Solid Edge part; units mm, degrees
sketch "Sketch1" plane through (0, 0, 0) normal (0, 0, 1) x (1, 0, 0)
  line L0 (0, 32.5) -> (0, 6.5)
  line L1 (13, 6.5) -> (13, 32.5)
  arc A0 (13, 6.5) -> (0, 6.5) centre (6.5, 6.5) cw
  arc A1 (0, 32.5) -> (13, 32.5) centre (6.5, 32.5) cw
extrude "Protrusion1" add sketch "Sketch1" along normal blind 6.5
sketch "Sketch2" plane through (6.5, 0, 0) normal (1, 0, 0) x (0, 1, 0)
  line L0 (3.5, 5.5) -> (3.5, 6.5)
  line L1 (3.5, 6.5) -> (6.5, 6.5)
  line L2 (6.5, 1) -> (6.5, 6.5)
  line L3 (3.5, 1) -> (6.5, 1)
  line L4 (3.5, 1) -> (2.6811, 3.25)
  line L5 (3.5, 5.5) -> (2.6811, 3.25)
revolve "RevolvedCutout1" cut sketch "Sketch2" angle 360 about axis through (6.5, 6.5, 1) along (0, 0, 1)
chamfer "Chaflán_38" distance 0.75 angle 45 1 edges at (6.5, 3.5, 6.5)
pattern_linear "Pattern1" count 3 spacing 13 along (0, 1, 0) of "RevolvedCutout1", "Chaflán_38"
chamfer "Chaflán_39" distance 1.5 angle 45 8 edges at (13, 19.5, 6.5) (6.5, 0, 6.5) (0, 19.5, 6.5) (6.5, 39, 6.5) (13, 19.5, 0) (6.5, 0, 0) (0, 19.5, 0) (6.5, 39, 0)
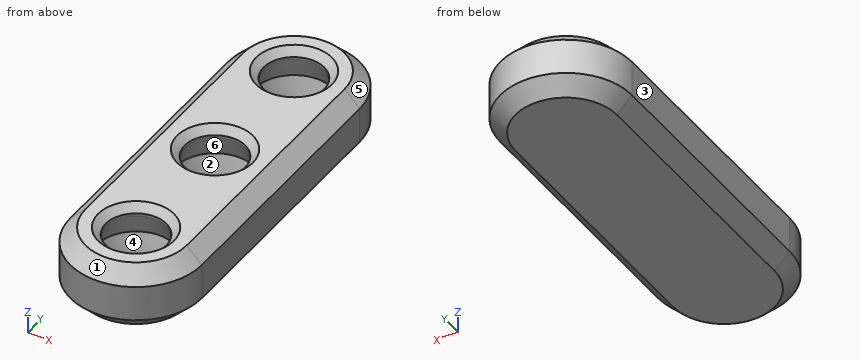
Can you work these out from the model? Positions are in its coordinate system, mm. Face numbers are marked on the shaded views. A direction names the side the tool comes from. Coordinates: 2 decimals unless noted, no trailing zeros. Write each loop counter-clockwise with the first axis right and the second up, starting at its lowest first coordinate (ties: lowest second). Pieces come first, ordered by that corner, then holes. Notation, with made-up numbers: M -29,-18 L 7,-18 A27 ccw 7,11 Z; hole C 55,69.25 d5. An arc over 180 degrees is marked long. Use one line per item in the form item = value.
Q1. I need wall thicknesses on line 1 along Y through (x, z) = (8.5, 4.5); line 2 along Y through (x, z) = (5.25, 6); line 3 along X through (y, z) = (32.5, 5.7). Which ranges of each line are inside material? Lowest first, please. Write a range as from..to.
Model answer:
line_1 = 0.32..3.8, 9.2..16.8, 22.2..29.8, 35.2..38.68
line_2 = 1.14..3.5, 9.5..16.5, 22.5..29.5, 35.5..37.86
line_3 = 0.7..3.5, 9.5..12.3
Q2. For P1, Ø3, axis at x = 5.5, y = 31, coming from the +Z side; P2, Ø3, axis at x = 4.5, z = 0.5, coming from the -Y side; P3, Ø1.8, axis at x = 6, y = 5, coming from the +Z side, each with a flat end and sliding along its axis, tell me the tip position at first contact or that it passes through.
Model answer:
P1 = 6.05
P2 = 0.06
P3 = 1
Q3. For the marked faces 5 and 6, which set-ups out of +Z, -Z, +X, -X, +Y, -Y let a thin tool reach every point of the face, with its end or its side?
Model answer:
face_5 = +Z, +Y
face_6 = none
Q4. If we section it at A-A (y = 19.5): Write out the boundary of the cut face in (x, z), then the cut area to 3 significant figures.
Model answer:
outline = M 0,1.5 L 1.5,0 L 11.5,0 L 13,1.5 L 13,5 L 11.5,6.5 L 10.25,6.5 L 9.5,5.75 L 9.5,5.5 L 10.32,3.25 L 9.5,1 L 3.5,1 L 2.68,3.25 L 3.5,5.5 L 3.5,5.75 L 2.75,6.5 L 1.5,6.5 L 0,5 Z
area = 42.8 mm^2
Q5. If we section it at B-B (z = 4.25): Write out the boundary of the cut face in (x, y).
Model answer:
outline = M 0,6.5 A6.5 ccw 13,6.5 L 13,32.5 A6.5 ccw 0,32.5 Z; hole C 6.5,6.5 d6.91; hole C 6.5,19.5 d6.91; hole C 6.5,32.5 d6.91
Q6. We'd pull the mould along Z, two halves only. Please class the marked faces 1, 2, 3 and 4: +Z half, -Z half, draft (parallel to the pull), parting line (faces both ways), or undercut.
Model answer:
face_1 = +Z half
face_2 = undercut
face_3 = draft
face_4 = undercut
Q7. If we section it at C-C (y = 28): Write out the boundary of the cut face in (x, z).
Model answer:
outline = M 0,1.5 L 1.5,0 L 11.5,0 L 13,1.5 L 13,5 L 11.5,6.5 L 1.5,6.5 L 0,5 Z
